Autodesk Inventor part; units mm, degrees
ref_plane "YZ Plane" through (0, 0, 0) normal (1, 0, 0) x (0, 1, 0)
ref_plane "XZ Plane" through (0, 0, 0) normal (0, 1, 0) x (-1, 0, 0)
ref_plane "XY Plane" through (0, 0, 0) normal (0, 0, 1) x (1, 0, 0)
sketch "Sketch1" plane through (0, 0, 0) normal (0, 1, 0) x (-1, 0, 0)
  line L0 (0, 0) -> (76.2, 0)
  line L1 (76.2, 0) -> (76.2, -152.4)
  line L2 (76.2, -152.4) -> (0, -152.4)
  line L3 (0, -152.4) -> (0, 0)
  dimension "d0" = 76.2
  dimension "d1" = 152.4
extrude "Extrusion1" add sketch "Sketch1" along normal blind 6.35
sketch "Sketch2" plane through (0, 6.35, 0) normal (0, 1, 0) x (1, 0, 0)
  line L0 (-76.2, 152.4) -> (-76.2, 0)
  line L1 (0, 0) -> (-76.2, 0)
  line L2 (-76.2, 0) -> (-76.2, 12.7)
  line L3 (-76.2, 12.7) -> (0, 12.7)
  line L4 (0, 12.7) -> (0, 0)
  dimension "d4" = 12.7
extrude "Extrusion2" add sketch "Sketch2" along normal blind 22.86
sketch "Sketch3" plane through (0, 29.21, 0) normal (0, 1, 0) x (1, 0, 0)
  line L0 (0, 152.4) -> (0, 0)
  line L1 (0, 12.7) -> (-76.2, 12.7)
  line L2 (-76.2, 12.7) -> (-76.2, -139.7)
  line L3 (-76.2, -139.7) -> (0, -139.7)
  line L4 (0, -139.7) -> (0, 12.7)
  line L5 (0, 12.7) -> (-76.2, 12.7)
  dimension "d7" = 76.2
  dimension "d8" = 152.4
extrude "Extrusion3" add sketch "Sketch3" along normal blind 50.8
sketch "Sketch4" plane through (-76.2, 0, -152.4) normal (-1, 0, 0) x (0, 0, 1)
  line L0 (292.1, 29.21) -> (152.4, 29.21)
  line L1 (152.4, 29.21) -> (292.1, 61.1529)
  line L2 (152.4, 0) -> (152.4, 29.21)
  line L3 (152.4, 29.21) -> (292.1, 29.21)
  line L4 (292.1, 29.21) -> (292.1, 80.01)
extrude "Extrusion4" cut sketch "Sketch4" against normal through all
properties part number "Pillow Holder"
The listing builds one solid part. Answer for the finished solid, in the listing's coordinates (mm). A direction names the side the tool comes from. Coordinates: 2 decimals unless noted, no trailing zeros. Order: outer loops, then holes, each group sorted by start corner. A loop starts at its lowest first (then second) coordinate and runs counter-clockwise, first axis right, second up. Notation, with made-up numbers: (18, -37.75) -> (37, -37.75) arc R26 ccw to (37, -14.75) -> close; hole circle Ø4 at (16, -39.5). An arc over 180 degrees is marked (long way). Answer in a Markdown table with one row per item. Add a question column.
Item 1: Which of the six approach directions +Z, -Z, +X, -X, +Y, -Y give full straight-line access (tool end or side, diameter ignored) to faces 1 (the face through (-39, 70, 139.7)), 2 (the face through (-38, 43, -12.7)), 3 (the face through (-38, 14, 0))?
Item 2: Each of these flat-tipped pins is pushed along its axis until it touches: P1, Ø1, axis at x = -52, y = 64, coming from the -Z side; P2, Ø3, axis at x = -32.5, y = 8.5, coming from the +Z side; P3, Ø4, axis at x = -25, z = -53, coming from the -Y side; P4, Ø5, axis at x = -31.5, z = -55.5, coming from the +Y side. Where does it stop, or does it pass through?
Item 3: Find section B-B (z = -106.5). Write down the section's boundary in (x, y).
Item 4: Find section C-C (y = 12.5). Write down the section's boundary in (x, z).
Item 5: Find the intervals of material crossed by L1, parallel to Y at x = -46, z = -28.5; L2, parallel to Z at x = -58, y = 23; L3, parallel to Z at x = -10, y = 4.5, in increasing order. Write a range as from..to.
Item 6: Find section A-A (x = -18). Write down the section's boundary in (y, z), then the cut area to 3 significant figures.
Result set:
| question | item | result |
|---|---|---|
| 1 | face 1 | +Z, +X, -X, +Y, -Y |
| 1 | face 2 | -Z, +X, -X, +Y |
| 1 | face 3 | +Z, +X, -X, -Y |
| 2 | P1 | stops at z = -12.7 |
| 2 | P2 | stops at z = 0 |
| 2 | P3 | stops at y = 0 |
| 2 | P4 | stops at y = 6.35 |
| 3 | outline | (-76.2, 0) -> (0, 0) -> (0, 6.35) -> (-76.2, 6.35) -> close |
| 4 | outline | (-76.2, -12.7) -> (0, -12.7) -> (0, 0) -> (-76.2, 0) -> close |
| 5 | L1 | y = 0..6.35 |
| 5 | L2 | z = -12.7..0 |
| 5 | L3 | z = -152.4..0 |
| 6 | outline | (0, -152.4) -> (6.35, -152.4) -> (6.35, -12.7) -> (80.01, -12.7) -> (80.01, 139.7) -> (61.15, 139.7) -> (29.21, 0) -> (0, 0) -> close |
| 6 | area | 6,770 mm² |
